from build123d import *

# Parameters (mm, degrees)
SKETCH_1_W             = 70
SKETCH_1_H             = 43
EXTRUDE_1_DEPTH        = 48.5
SKETCH_2_W             = 50
SKETCH_2_H             = 27
SKETCH_2_H_2           = 8
SKETCH_2_W_2           = 10
CUT_EXTRUDE_1_DEPTH    = 40
HOLE_WIZARD_M3_1_D     = 2.5
HOLE_WIZARD_M3_1_DEPTH = 15
HOLE_WIZARD_M3_1_TIP   = 0.751075774


with BuildPart() as part:
    # 草图1 → 凸台-拉伸1 (new body)
    with BuildSketch(Plane.XY):
        Rectangle(SKETCH_1_W, SKETCH_1_H)
    extrude(amount=EXTRUDE_1_DEPTH)

    # 草图2 → 切除-拉伸1 (cut)
    with BuildSketch(Plane(origin=(0, 0, 0), x_dir=(-1, 0, 0), z_dir=(0, 0, -1))):
        Rectangle(SKETCH_2_W, SKETCH_2_H)
        with Locations((0, -17.5)):
            Rectangle(SKETCH_2_W, SKETCH_2_H_2)
        with Locations((-30, 0)):
            Rectangle(SKETCH_2_W_2, SKETCH_2_H)
        with Locations((0, 17.5)):
            Rectangle(SKETCH_2_W, SKETCH_2_H_2)
        with Locations((30, 0)):
            Rectangle(SKETCH_2_W_2, SKETCH_2_H)
    extrude(amount=-CUT_EXTRUDE_1_DEPTH, mode=Mode.SUBTRACT)

    # M3 螺纹孔1
    with Locations(Plane(origin=(0, 0, 0), x_dir=(-1, 0, 0), z_dir=(0, 0, -1))):
        with Locations((-30, 17.5), (30, 17.5), (30, -17.5), (-30, -17.5)):
            Hole(HOLE_WIZARD_M3_1_D / 2, depth=HOLE_WIZARD_M3_1_DEPTH)
            with Locations((0, 0, -(HOLE_WIZARD_M3_1_DEPTH + HOLE_WIZARD_M3_1_TIP / 2))):  # 118° drill point
                Cone(0, HOLE_WIZARD_M3_1_D / 2, HOLE_WIZARD_M3_1_TIP, mode=Mode.SUBTRACT)


solid = part.part
For this review, take the finished solid that the model builds, in its own axes (mm). A direction names the side the tool comes from. Give positions to 0.01 mm unless a question says otherwise; leave off trailing zeros. Write each loop counter-clockwise with the first axis right and the second up, starting at its lowest first coordinate (ties: lowest second). Pieces come first, ordered by that corner, then holes. Notation, with made-up numbers: (49, -10) -> (80, -10) arc R28 cw to (80, 29) -> close; hole circle Ø4 at (48, 78). An arc over 180 degrees is marked (long way). Use CSV: the item, a comma, the result in double quotes.
Q1. Take a section at D-D, the plane y = -2. Write out the cut boundary in (x, z).
Conclusion:
outline,"(-35, 40) -> (35, 40) -> (35, 48.5) -> (-35, 48.5) -> close"
Q2. To check wall thickness, follow probe 1 along Y at (x, z) = (30, 11); probe 2 along X at (y, z) = (-17.5, 3.5); probe 3 along Z at (x, y) = (-30, -11.5). State the ranges of each line that lie inside material, in increasing order. Write a range as [from, to].
Conclusion:
probe 1,"[-21.5, -18.75], [-16.25, -13.5], [13.5, 16.25], [18.75, 21.5]"
probe 2,"[-35, -31.25], [-28.75, -25], [25, 28.75], [31.25, 35]"
probe 3,"[40, 48.5]"
Q3. Take a section at C-C, the plane x = -26. Write out the cut boundary in (y, z), then the cut area to 3 significant figures.
Conclusion:
outline,"(-21.5, 0) -> (-13.5, 0) -> (-13.5, 40) -> (13.5, 40) -> (13.5, 0) -> (21.5, 0) -> (21.5, 48.5) -> (-21.5, 48.5) -> close"
area,"1,010 mm2"
Q4. Take a section at B-B, the plane z = 17. Write out the cut boundary in (x, y).
Conclusion:
outline,"(-35, -21.5) -> (-25, -21.5) -> (-25, -13.5) -> (-35, -13.5) -> close; (-35, 13.5) -> (-25, 13.5) -> (-25, 21.5) -> (-35, 21.5) -> close; (25, -21.5) -> (35, -21.5) -> (35, -13.5) -> (25, -13.5) -> close; (25, 13.5) -> (35, 13.5) -> (35, 21.5) -> (25, 21.5) -> close"
Q5. For P1, Ø10, axis at y = -11.5, z = 34, coming from the +X side; P2, Ø2, axis at x = -30, y = 17.5, coming from the -Z side; P3, Ø13, axis at x = -9.5, y = 6, coming from the -Z side, all flat-tipped, find the tip position at first contact; note any pin that passes through.
Conclusion:
P1,"x = 35"
P2,"z = 15.15"
P3,"z = 40"
Q6. Tool access review of faces 4 (the face through (31.04, 18.44, 0)), 5 (the face through (0, -21.5, 45)), 6 (the face through (-25, -18, 20)), 7 (the face through (0, 0, 40)), 8 (the face through (-30, 13.5, 20)): name each direction out of +Z, -Z, +X, -X, +Y, -Y from which nothing blocks a thin tool from reaching the whole face with its end or side.
Conclusion:
face 4,"-Z, +X, -X, +Y, -Y"
face 5,"+Z, -Z, +X, -X, -Y"
face 6,"-Z, +Y, -Y"
face 7,"-Z"
face 8,"-Z, +X, -X"
Q7. Mouldability with a two-part tool opening along X and no side actions: class faces 1 (the face through (29.8, -17.58, 15.62)), 2 (the face through (30, -13.5, 20)), 3 (the face through (35, -15, 29)) as pulls with the +X half, pulls with the -X half, needs draft (parallel to the pull), parting line crosses it, or undercut.
Conclusion:
face 1,"undercut"
face 2,"needs draft"
face 3,"pulls with the +X half"
Q8. Take a section at A-A, the plane z = 10. Write out the cut boundary in (x, y).
Conclusion:
outline,"(-35, -21.5) -> (-25, -21.5) -> (-25, -13.5) -> (-35, -13.5) -> close; (-35, 13.5) -> (-25, 13.5) -> (-25, 21.5) -> (-35, 21.5) -> close; (25, -21.5) -> (35, -21.5) -> (35, -13.5) -> (25, -13.5) -> close; (25, 13.5) -> (35, 13.5) -> (35, 21.5) -> (25, 21.5) -> close; hole circle Ø2.5 at (-30, -17.5); hole circle Ø2.5 at (-30, 17.5); hole circle Ø2.5 at (30, -17.5); hole circle Ø2.5 at (30, 17.5)"
